```python
from build123d import *

# Parameters (mm, degrees)
F0_W     = 56.6928
F0_H     = 42.1894
F1_DEPTH = 25.4
F3_D     = 6.35


with BuildPart() as f1:
    # F0 (on Top) → F1 (new body)
    with BuildSketch(Plane.XY):
        with Locations((28.3464, 21.0947)):
            Rectangle(F0_W, F0_H)
    extrude(amount=F1_DEPTH)

    # F3 (through all)
    with Locations(Plane.XY.offset(25.4)):
        with Locations((9.525, 9.525), (9.525, 32.6644), (47.1678, 32.6644), (47.1678, 9.525)):
            Hole(F3_D / 2)


solid = f1.part
```
CAD build for the part. Positions are in the model's coordinates, mm. Give positions to 0.01 mm unless a question says otherwise; leave off trailing zeros. Order: outer loops, then holes, each group sorted by start corner. A loop starts at its lowest first (then second) coordinate and runs counter-clockwise, first axis right, second up.
(1) Saw through at A-A, the plane x = 11.5. Give the cut face in (y, z), then the cut area to 3 significant figures.
(2) Mould opens along Y. For faces 1 (the flat face through (28, 21, 25.4)), 2 (the flat face through (28, 0, 13)), 3 (the cylindrical face through (50.34, 32.8, 12.52)) say: released by +Y, released by -Y, zero draft, split by the parting line, or undercut.
(3) Saw through at C-C, the plane x = 45. Give the cut face in (y, z).
(4) Saw through at B-B, the plane z = 7.25. Give the cut face in (x, y) (3 decimals).
(5) Drill centre lines: L1, parallel to Y at x = 47, z = 24.75; L2, parallel to X at y = 8, z = 7.5; L3, parallel to X at y = 7, z = 5. Where is each one in solid material? Low to high.
Results found:
1. outline: (0, 0) - (7.04, 0) - (7.04, 25.4) - (0, 25.4) - close; (12.01, 0) - (30.18, 0) - (30.18, 25.4) - (12.01, 25.4) - close; (35.15, 0) - (42.19, 0) - (42.19, 25.4) - (35.15, 25.4) - close
1. area: 819 mm2
2. face 1: zero draft
2. face 2: released by -Y
2. face 3: undercut
3. outline: (0, 0) - (7.21, 0) - (7.21, 25.4) - (0, 25.4) - close; (11.84, 0) - (30.34, 0) - (30.34, 25.4) - (11.84, 25.4) - close; (34.98, 0) - (42.19, 0) - (42.19, 25.4) - (34.98, 25.4) - close
4. outline: (0, 0) - (56.693, 0) - (56.693, 42.189) - (0, 42.189) - close; hole circle Ø6.35 at (9.525, 9.525); hole circle Ø6.35 at (9.525, 32.664); hole circle Ø6.35 at (47.168, 9.525); hole circle Ø6.35 at (47.168, 32.664)
5. L1: y = 0 to 6.35, 12.7 to 29.49, 35.83 to 42.19
5. L2: x = 0 to 6.74, 12.31 to 44.38, 49.95 to 56.69
5. L3: x = 0 to 7.6, 11.45 to 45.24, 49.09 to 56.69
